Here's how the part is built. I have some questions about the finished solid (model axes, mm). A direction names the side the tool comes from. Give positions to 0.01 mm unless a question says otherwise; leave off trailing zeros. Write each question's results on one line, items separated by ' | '. Start each with the question number.
Item 1: Please list where these lines run through material, in increasing order: line 1 along X through (y, z) = (4.25, -39); line 2 along X through (y, z) = (9.75, 49.5); line 3 along X through (y, z) = (10, -20).
Item 2: Will these pins go through, and if not, where does the flat tip stop? P1, Ø3, axis at x = -41, y = 4.5, coming from the -Z side; P2, Ø6.5, axis at x = 38.17, z = 38.17, coming from the -Y side; P3, Ø6, axis at y = 16, z = 12.5, coming from the +X side; P4, Ø9, axis at x = 16, z = 19, coming from the +Y side (3 decimals).
Item 3: Which directions (+Z, -Z, +X, -X, +Y, -Y) give clear straight access to the entire face, cutting with the end or side of a thin tool? Please do faces 1 (the cylindrical face through (-22.36, 12.22, -14.69)), 2 (the cylindrical face through (19.73, 5.14, -20.36)).
Item 4: We'd pull the mould along X, two halves only. Please class faces 3 (the cylindrical face through (40.29, 14.13, 43.3)), 4 (the cylindrical face through (-40.18, 8.77, -52.41)), 5 (the flat face through (-14, 0, 14)): +X half, -X half, draft (parallel to the pull), parting line (faces both ways), or undercut.
Item 5: Suppose I cut it at A-A on y = 13.25. Count the separate pieces of the cut face and the enclosed holes in it, then the cut area to 3 significant figures.
```python
from build123d import *

# Parameters (mm, degrees)
SKETCH1_R                                     = 66.04
BOSS_EXTRUDE1_DEPTH                           = 17.78
SKETCH2_R                                     = 36.4998
CUT_EXTRUDE1_DEPTH                            = 1.905
CUT_EXTRUDE2_DEPTH                            = 95.734253705
CUT_EXTRUDE2_DEPTH_BACK                       = 19.05
SKETCH3_R                                     = 17.78
F_1_4_20_TAPPED_HOLE1_AT_2_COUNT              = 2
F_1_4_20_TAPPED_HOLE1_AT_2_PITCH              = 69.596984938
F_1_4_20_TAPPED_HOLE1_AT_3_COUNT              = 2
F_1_4_20_TAPPED_HOLE1_AT_3_PITCH              = 98.425
F_1_4_20_TAPPED_HOLE1_AT_4_COUNT              = 2
F_1_4_20_TAPPED_HOLE1_AT_4_PITCH              = 69.596984938
CBORE_FOR_1_4_SOCKET_HEAD_CAP_SCREW1_AT_COUNT = 2
CBORE_FOR_1_4_SOCKET_HEAD_CAP_SCREW1_AT_PITCH = 25
CBORE_FOR_1_4_SOCKET_HEAD_CAP_SCREW1_2_COUNT  = 2
CBORE_FOR_1_4_SOCKET_HEAD_CAP_SCREW1_2_PITCH  = 25
CBORE_FOR_1_4_SOCKET_HEAD_CAP_SCREW1_3_COUNT  = 2
CBORE_FOR_1_4_SOCKET_HEAD_CAP_SCREW1_3_PITCH  = 25
CBORE_FOR_1_4_SOCKET_HEAD_CAP_SCREW1_4_COUNT  = 2
CBORE_FOR_1_4_SOCKET_HEAD_CAP_SCREW1_4_PITCH  = 25
CHAMFER1_SIZE                                 = 0.381
CBORE_FOR_1_4_SOCKET_HEAD_CAP_SCREW2_AT_COUNT = 2
CBORE_FOR_1_4_SOCKET_HEAD_CAP_SCREW2_AT_PITCH = 53.975
CBORE_FOR_1_4_SOCKET_HEAD_CAP_SCREW2_2_COUNT  = 2
CBORE_FOR_1_4_SOCKET_HEAD_CAP_SCREW2_2_PITCH  = 53.975
CBORE_FOR_1_4_SOCKET_HEAD_CAP_SCREW2_3_COUNT  = 2
CBORE_FOR_1_4_SOCKET_HEAD_CAP_SCREW2_3_PITCH  = 53.975
CBORE_FOR_1_4_SOCKET_HEAD_CAP_SCREW2_4_COUNT  = 2
CBORE_FOR_1_4_SOCKET_HEAD_CAP_SCREW2_4_PITCH  = 53.975


with BuildPart() as part:
    # Sketch1 → Boss-Extrude1 (new body)
    with BuildSketch(Plane(origin=(0, 0, 0), x_dir=(1, 0, 0), z_dir=(0, 1, 0))):
        with Locations(Location((0, 0, 0), (0, 0, 270))):
            Circle(SKETCH1_R)
    extrude(amount=BOSS_EXTRUDE1_DEPTH)

    # Sketch2 → Cut-Extrude1 (cut)
    with BuildSketch(Plane(origin=(0, 17.78, 0), x_dir=(1, 0, 0), z_dir=(0, 1, 0))):
        with Locations(Location((0, 0, 0), (0, 0, 270))):
            Circle(SKETCH2_R)
    extrude(amount=-CUT_EXTRUDE1_DEPTH, mode=Mode.SUBTRACT)

    # Sketch3 → Cut-Extrude2 (cut, two sides: drawn at the far end of the back side and taken through both)
    with BuildSketch(Plane(origin=(0, 15.875, 0), x_dir=(1, 0, 0), z_dir=(0, 1, 0)).offset(-CUT_EXTRUDE2_DEPTH_BACK)):
        with Locations(Location((0, 0, 0), (0, 0, 270))):
            Circle(SKETCH3_R)
    extrude(amount=CUT_EXTRUDE2_DEPTH + CUT_EXTRUDE2_DEPTH_BACK, mode=Mode.SUBTRACT)

    # Sketch5 → 1/4-20 Tapped Hole1 (revolve, cut)
    with BuildSketch(Plane(origin=(0, 17.78, -49.2125), x_dir=(0, 0, 1), z_dir=(1, 0, 0))):
        Polygon((0, 0), (0, 17.78), (3.1877, 17.78), (2.5527, 17.145), (2.5527, 0.635), (3.1877, 0), align=None)
    f_1_4_20_tapped_hole1 = revolve(axis=Axis((0, 24.13, -49.2125), (0, -1, 0)), mode=Mode.SUBTRACT)

    # 1/4-20 Tapped Hole1 at 2: 1/4-20 Tapped Hole1 ×2
    with Locations(*[Vector(0.7071067811865476, 0, 0.7071067811865476) * (i * F_1_4_20_TAPPED_HOLE1_AT_2_PITCH) for i in range(1, F_1_4_20_TAPPED_HOLE1_AT_2_COUNT)]):
        add(f_1_4_20_tapped_hole1, mode=Mode.SUBTRACT)

    # 1/4-20 Tapped Hole1 at 3: 1/4-20 Tapped Hole1 ×2
    with Locations(*[(0, 0, i * F_1_4_20_TAPPED_HOLE1_AT_3_PITCH) for i in range(1, F_1_4_20_TAPPED_HOLE1_AT_3_COUNT)]):
        add(f_1_4_20_tapped_hole1, mode=Mode.SUBTRACT)

    # 1/4-20 Tapped Hole1 at 4: 1/4-20 Tapped Hole1 ×2
    with Locations(*[Vector(-0.7071067811865476, 0, 0.7071067811865476) * (i * F_1_4_20_TAPPED_HOLE1_AT_4_PITCH) for i in range(1, F_1_4_20_TAPPED_HOLE1_AT_4_COUNT)]):
        add(f_1_4_20_tapped_hole1, mode=Mode.SUBTRACT)

    # Sketch7 → CBORE for 1/4 Socket Head Cap Screw1 (revolve, cut)
    with BuildSketch(Plane(origin=(0, 15.875, 0), x_dir=(0, 0, 1), z_dir=(1, 0, 0))):
        Polygon((0, 0), (0, 15.875), (4.0132, 15.875), (3.3782, 15.24), (3.3782, 6.35), (5.55625, 6.35), (5.55625, 1.03251), (6.58876, 0), align=None)
    cbore_for_1_4_socket_head_cap_screw1 = revolve(axis=Axis((0, 22.225, 0), (0, -1, 0)), mode=Mode.SUBTRACT)

    # CBORE for 1/4 Socket Head Cap Screw1 at: CBORE for 1/4 Socket Head Cap Screw1 ×2
    with Locations(*[Vector(0.7071067811865476, 0, -0.7071067811865476) * (i * CBORE_FOR_1_4_SOCKET_HEAD_CAP_SCREW1_AT_PITCH) for i in range(1, CBORE_FOR_1_4_SOCKET_HEAD_CAP_SCREW1_AT_COUNT)]):
        add(cbore_for_1_4_socket_head_cap_screw1, mode=Mode.SUBTRACT)

    # CBORE for 1_4 Socket Head Cap Screw1 2: CBORE for 1/4 Socket Head Cap Screw1 ×2
    with Locations(*[Vector(-0.7071067811865476, 0, 0.7071067811865476) * (i * CBORE_FOR_1_4_SOCKET_HEAD_CAP_SCREW1_2_PITCH) for i in range(1, CBORE_FOR_1_4_SOCKET_HEAD_CAP_SCREW1_2_COUNT)]):
        add(cbore_for_1_4_socket_head_cap_screw1, mode=Mode.SUBTRACT)

    # CBORE for 1_4 Socket Head Cap Screw1 3: CBORE for 1/4 Socket Head Cap Screw1 ×2
    with Locations(*[Vector(-0.7071067811865475, 0, -0.7071067811865477) * (i * CBORE_FOR_1_4_SOCKET_HEAD_CAP_SCREW1_3_PITCH) for i in range(1, CBORE_FOR_1_4_SOCKET_HEAD_CAP_SCREW1_3_COUNT)]):
        add(cbore_for_1_4_socket_head_cap_screw1, mode=Mode.SUBTRACT)

    # CBORE for 1_4 Socket Head Cap Screw1 4: CBORE for 1/4 Socket Head Cap Screw1 ×2
    with Locations(*[Vector(0.7071067811865477, 0, 0.7071067811865475) * (i * CBORE_FOR_1_4_SOCKET_HEAD_CAP_SCREW1_4_PITCH) for i in range(1, CBORE_FOR_1_4_SOCKET_HEAD_CAP_SCREW1_4_COUNT)]):
        add(cbore_for_1_4_socket_head_cap_screw1, mode=Mode.SUBTRACT)

    # Chamfer1
    chamfer1_edges = [part.edges().sort_by_distance(p)[0] for p in [
        (0, 15.875, -17.78),
        (0, 0, -17.78),
        (0, 0, -66.04),
        (0, 17.78, -66.04),
        (0, 17.78, -36.4998),
    ]]
    chamfer(chamfer1_edges, length=CHAMFER1_SIZE)

    # Sketch9 → CBORE for 1/4 Socket Head Cap Screw2 (revolve, cut)
    with BuildSketch(Plane(origin=(0, 17.78, 0), x_dir=(0, 0, 1), z_dir=(1, 0, 0))):
        Polygon((0, 0), (0, 17.78), (4.0132, 17.78), (3.3782, 17.145), (3.3782, 6.35), (5.55625, 6.35), (5.55625, 1.03251), (6.58876, 0), align=None)
    cbore_for_1_4_socket_head_cap_screw2 = revolve(axis=Axis((0, 24.13, 0), (0, -1, 0)), mode=Mode.SUBTRACT)

    # CBORE for 1/4 Socket Head Cap Screw2 at: CBORE for 1/4 Socket Head Cap Screw2 ×2
    with Locations(*[Vector(0.7071067811865476, 0, 0.7071067811865475) * (i * CBORE_FOR_1_4_SOCKET_HEAD_CAP_SCREW2_AT_PITCH) for i in range(1, CBORE_FOR_1_4_SOCKET_HEAD_CAP_SCREW2_AT_COUNT)]):
        add(cbore_for_1_4_socket_head_cap_screw2, mode=Mode.SUBTRACT)

    # CBORE for 1_4 Socket Head Cap Screw2 2: CBORE for 1/4 Socket Head Cap Screw2 ×2
    with Locations(*[Vector(-0.7071067811865476, 0, -0.7071067811865476) * (i * CBORE_FOR_1_4_SOCKET_HEAD_CAP_SCREW2_2_PITCH) for i in range(1, CBORE_FOR_1_4_SOCKET_HEAD_CAP_SCREW2_2_COUNT)]):
        add(cbore_for_1_4_socket_head_cap_screw2, mode=Mode.SUBTRACT)

    # CBORE for 1_4 Socket Head Cap Screw2 3: CBORE for 1/4 Socket Head Cap Screw2 ×2
    with Locations(*[Vector(-0.7071067811865477, 0, 0.7071067811865475) * (i * CBORE_FOR_1_4_SOCKET_HEAD_CAP_SCREW2_3_PITCH) for i in range(1, CBORE_FOR_1_4_SOCKET_HEAD_CAP_SCREW2_3_COUNT)]):
        add(cbore_for_1_4_socket_head_cap_screw2, mode=Mode.SUBTRACT)

    # CBORE for 1_4 Socket Head Cap Screw2 4: CBORE for 1/4 Socket Head Cap Screw2 ×2
    with Locations(*[Vector(0.7071067811865475, 0, -0.7071067811865477) * (i * CBORE_FOR_1_4_SOCKET_HEAD_CAP_SCREW2_4_PITCH) for i in range(1, CBORE_FOR_1_4_SOCKET_HEAD_CAP_SCREW2_4_COUNT)]):
        add(cbore_for_1_4_socket_head_cap_screw2, mode=Mode.SUBTRACT)


solid = part.part
```
Checked values:
1) line 1: x = -53.29 to -41.44, -34.89 to 34.89, 41.44 to 53.29 | line 2: x = -43.72 to -2.54, 2.54 to 43.72 | line 3: x = -62.94 to -22.73, -12.63 to 12.63, 22.73 to 62.94
2) P1: stops at z = -52.92 | P2: passes through | P3: stops at x = 65.35 | P4: stops at y = 15.875
3) face 1: +Y | face 2: +Y, -Y
4) face 3: undercut | face 4: parting line | face 5: draft
5) separate pieces: 1 | enclosed holes: 13 | area: 11,900 mm^2
